Input: part model. Units: mm. Frame: model coordinates. A direction names the side the tool comes from. Give positions to 0.01 mm unless a question says otherwise; leave off trailing zeros. Write each loop counter-clockwise with the first axis right and the second up, starting at its lowest first coordinate (ties: lowest second). Pieces come first, ordered by that corner, then holes. Notation, with made-up numbers: (54, 10.5) - (103, 10.5) arc R16 ccw to (103, 32.5) - close; hole circle Ø2 at (-13, 88.5). An arc over 180 degrees is marked (long way). Use a Markdown table: item, result. Add a question column.
1. Section query D-D, the plane x = 49. Return loops of the section in (y, z), plus the area to 3 significant figures.
2. Section query C-C, the plane z = 49.5. Return loops of the section in (x, y).
3. Section query B-B, the plane y = 0. Return loops of the section in (x, z), plus the area to 3 significant figures.
4. Material intervals for probe 1 along Y at (x, z) = (47.8, 6.5); probe 2 along Y at (x, z) = (-47.8, 45); probe 3 along X at (y, z) = (-7, 34), sorted ascending.
5. Mould query, pull axis Y, two halves, no side actions, for faces 3 (the flat face through (-1, -57.6, 44)), 4 (the cylindrical face through (37.177, -4.405, 49.36)), 5 (the flat face through (-43, 0, 8.8)), 6 (the flat face through (-1, 1, 88.8)). Classes: released by +Y, released by -Y, zero draft, split by the parting line, or undercut.
6. Set-up query: faces 1 (the cylindrical face through (-36.83, 3.45, 49.36)), 2 (the flat face through (77.8, -1, 44)). Return all of +Z, -Z, +X, -X, +Y, -Y with unobstructed straight access to the full face (end or side cutting, diameter ignored); none if empty.
7. Section query A-A, the plane x = -47.8. Return loops of the section in (y, z).
```python
from build123d import *

# Parameters (mm, degrees)
SKIZZE1_W                                           = 155.6
SKIZZE1_H                                           = 115.2
AUFSATZ_LINEAR_AUSTRAGEN1_DEPTH                     = 88.8
STIRNSENKUNG_F_R_M8_SENKSCHRAUBE_KOPF_B_D           = 9
STIRNSENKUNG_F_R_M8_SENKSCHRAUBE_KOPF_B_CBORE_D     = 23
STIRNSENKUNG_F_R_M8_SENKSCHRAUBE_KOPF_B_CBORE_DEPTH = 80


with BuildPart() as part:
    # Skizze1 → Aufsatz-Linear austragen1 (new body)
    with BuildSketch(Plane.XY):
        Rectangle(SKIZZE1_W, SKIZZE1_H)
    extrude(amount=AUFSATZ_LINEAR_AUSTRAGEN1_DEPTH)

    # Stirnsenkung für M8 Senkschraube (Kopf Button)1 (through all)
    with Locations(Plane.XY.offset(88.8)):
        with Locations((-47.8, 0)):
            stirnsenkung_f_r_m8_senkschraube_kopf_b = CounterBoreHole(STIRNSENKUNG_F_R_M8_SENKSCHRAUBE_KOPF_B_D / 2, STIRNSENKUNG_F_R_M8_SENKSCHRAUBE_KOPF_B_CBORE_D / 2, STIRNSENKUNG_F_R_M8_SENKSCHRAUBE_KOPF_B_CBORE_DEPTH)

    # Spiegeln1: Stirnsenkung für M8 Senkschraube (Kopf Button)1 across plane
    add(stirnsenkung_f_r_m8_senkschraube_kopf_b.mirror(Plane(origin=(0, 0, 0), x_dir=(0, 0, 1), z_dir=(1, 0, 0))), mode=Mode.SUBTRACT)


solid = part.part
```
Result sheet:
| question | item | result |
|---|---|---|
| 1 | outline | (-57.6, 0) - (-4.34, 0) - (-4.34, 8.8) - (-11.44, 8.8) - (-11.44, 88.8) - (-57.6, 88.8) - close; (4.34, 0) - (57.6, 0) - (57.6, 88.8) - (11.44, 88.8) - (11.44, 8.8) - (4.34, 8.8) - close |
| 1 | area | 8,320 mm² |
| 2 | outline | (-77.8, -57.6) - (77.8, -57.6) - (77.8, 57.6) - (-77.8, 57.6) - close; hole circle Ø23 at (-47.8, 0); hole circle Ø23 at (47.8, 0) |
| 3 | outline | (-77.8, 0) - (-52.3, 0) - (-52.3, 8.8) - (-59.3, 8.8) - (-59.3, 88.8) - (-77.8, 88.8) - close; (-43.3, 0) - (43.3, 0) - (43.3, 8.8) - (36.3, 8.8) - (36.3, 88.8) - (-36.3, 88.8) - (-36.3, 8.8) - (-43.3, 8.8) - close; (52.3, 0) - (77.8, 0) - (77.8, 88.8) - (59.3, 88.8) - (59.3, 8.8) - (52.3, 8.8) - close |
| 3 | area | 9,980 mm² |
| 4 | probe 1 | y = -57.6 to -4.5, 4.5 to 57.6 |
| 4 | probe 2 | y = -57.6 to -11.5, 11.5 to 57.6 |
| 4 | probe 3 | x = -77.8 to -56.92, -38.68 to 38.68, 56.92 to 77.8 |
| 5 | face 3 | released by -Y |
| 5 | face 4 | undercut |
| 5 | face 5 | undercut |
| 5 | face 6 | zero draft |
| 6 | face 1 | +Z |
| 6 | face 2 | +Z, -Z, +X, +Y, -Y |
| 7 | outline | (-57.6, 0) - (-4.5, 0) - (-4.5, 8.8) - (-11.5, 8.8) - (-11.5, 88.8) - (-57.6, 88.8) - close; (4.5, 0) - (57.6, 0) - (57.6, 88.8) - (11.5, 88.8) - (11.5, 8.8) - (4.5, 8.8) - close |
